Part model, mm, in its own coordinate system. A direction names the side the tool comes from. Give positions to 0.01 mm unless a question says otherwise; leave off trailing zeros. Write each loop counter-clockwise with the first axis right and the second up, starting at its lowest first coordinate (ties: lowest second). Pieces come first, ordered by that corner, then holes. Notation, with made-up numbers: M 80.25,73 L 137.25,73 A17 cw 137.25,102 Z; hole C 68,65 d10. An arc over 180 degrees is marked long. Answer as CSV lines item,"result". Start each with the question number.
Item 1: Band-saw the part on A-A, the plane z = 0. List the corners of the cut face in (x, y).
Item 2: 3-axis set-ups, long thin cutter, end or side, ignore diameter. For faces 1 (the flat face through (1, 17, 14.39)), 2 (the flat face through (1, 15, 7)), 3 (the flat face through (14, 0, 7)): which of +Z, -Z, +X, -X, +Y, -Y reach the whole face in a straight line?
Item 3: Band-saw the part on B-B, the plane y = 3.25. List the corners of the cut face in (x, z).
Item 4: Band-saw the part on C-C, the plane x = 10. List the corners of the cut face in (y, z), then the cut area to 3 significant figures.
Item 5: Wall check: L1, parallel to X at y = 10.5, z = 14.75; L2, parallel to Y at x = -4.25, z = -5.5; L3, parallel to Y at x = -3, z = 1.75. Give the ranges that are in metal, low to high. Write a range as from..to.
Item 6: Two-plate mould, pull along Z, no slides. Class faces 4 (the flat face through (-11.475, 7, 8)), 5 (the flat face through (1, 17, 0.39)), 6 (the flat face through (-1.1, 15.4, -7.61)): +Z half, -Z half, draft (parallel to the pull), parting line (faces both ways), or undercut.
Item 7: Pin check, flat tips, straight feed: pin 1 (10 mm diameter, centred on x = 1.5, z = 11, fed in from -Y); pin 2 (5 mm diameter, centred on x = 4.5, z = 5.5, fed in from +Y). Stop position of each tip, or through.
from build123d import *

# Parameters (mm, degrees)
SKETCH1_W             = 1.5
SKETCH1_H             = 30
BOSS_EXTRUDE1_DEPTH   = 15
BOSS_EXTRUDE1_2_DEPTH = 15
SKETCH4_W             = 28
SKETCH4_H             = 30
BOSS_EXTRUDE2_DEPTH   = 1.5
SKETCH5_W             = 28
SKETCH5_H             = 8
BOSS_EXTRUDE3_DEPTH   = 2


with BuildPart() as part:
    # Sketch1 → Boss-Extrude1 (new body)
    with BuildSketch(Plane(origin=(0, 0, 0), x_dir=(1, 0, 0), z_dir=(0, 1, 0))):
        with Locations((-12.224763407, -7.389589905)):
            Rectangle(SKETCH1_W, SKETCH1_H)
    extrude(amount=BOSS_EXTRUDE1_DEPTH)



with BuildPart() as body_2:
    # Sketch1 → Boss-Extrude1 2 (new body)
    with BuildSketch(Plane(origin=(0, 0, 0), x_dir=(1, 0, 0), z_dir=(0, 1, 0))):
        with Locations((14.275236593, -7.389589905)):
            Rectangle(SKETCH1_W, SKETCH1_H)
    extrude(amount=BOSS_EXTRUDE1_2_DEPTH)


with BuildPart() as part_1:
    add(part.part)

    add(body_2.part)  # Boss-Extrude2 merges body 2
    # Sketch4 → Boss-Extrude2 (add)
    with BuildSketch(Plane(origin=(0, 15, 0), x_dir=(1, 0, 0), z_dir=(0, 1, 0))):
        with Locations((1.025236593, -7.389589905)):
            Rectangle(SKETCH4_W, SKETCH4_H)
    extrude(amount=BOSS_EXTRUDE2_DEPTH)

    # Sketch5 → Boss-Extrude3 (add)
    with BuildSketch(Plane(origin=(0, 16.5, 0), x_dir=(1, 0, 0), z_dir=(0, 1, 0))):
        with Locations((1.025236593, 3.610410095)):
            Rectangle(SKETCH5_W, SKETCH5_H)
        with Locations((1.025236593, -18.389589905)):
            Rectangle(SKETCH5_W, SKETCH5_H)
    extrude(amount=BOSS_EXTRUDE3_DEPTH)


solid = part_1.part
Output:
1,outline,"M -12.97,0 L -11.47,0 L -11.47,15 L 13.53,15 L 13.53,0 L 15.03,0 L 15.03,18.5 L -12.97,18.5 Z"
2,face 1,"+X, -X, +Y"
2,face 2,"+Z, -Z, -Y"
2,face 3,"+Z, -Z, +X, -X, -Y"
3,outline,"M -12.97,-7.61 L -11.47,-7.61 L -11.47,22.39 L -12.97,22.39 Z; M 13.53,-7.61 L 15.03,-7.61 L 15.03,22.39 L 13.53,22.39 Z"
4,outline,"M 15,-7.61 L 18.5,-7.61 L 18.5,0.39 L 16.5,0.39 L 16.5,14.39 L 18.5,14.39 L 18.5,22.39 L 15,22.39 Z"
4,area,"77.0 mm²"
5,L1,"-12.97..-11.47, 13.53..15.03"
5,L2,"15..18.5"
5,L3,"15..16.5"
6,face 4,"draft"
6,face 5,"undercut"
6,face 6,"-Z half"
7,pin 1,"y = 15"
7,pin 2,"y = 16.5"
